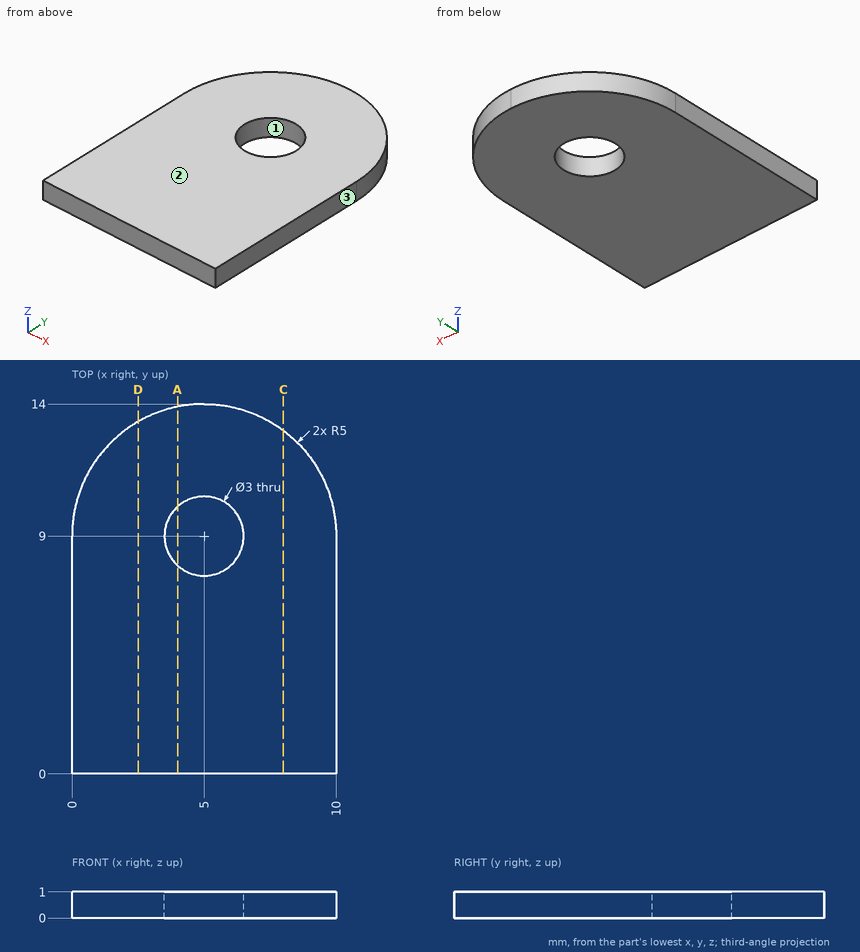
Study the drawing (mm; zero at the part's minimum x, y, z) and answer. Coordinates: 2 decimals unless noted, no trailing zeros. Loops run counter-clockwise (first coordinate to the right, second up) from the corner with the lowest first, then second, coordinate; pieces in that order, holes last. Notation, with made-up numbers: (20.25, 19) -> (63.25, 19) arc R12 cw to (63.25, 40) -> close; hole circle Ø3 at (42, 11). An arc over 180 degrees is marked (long way). Answer in a Markdown table with one row per item. Add a question column.
1. The part is cut by section A-A, the plane x = 4. Write down the section's boundary in (y, z).
2. The part is cut by section D-D, the plane x = 2.5. Write down the section's boundary in (y, z).
3. A flat-ended cylindrical pin translates along its axis: P1, Ø1.8, axis at x = 5, y = 9, coming from the -Z side. Find the tip coordinate at first contact, or state that the pin passes through.
4. Determine the mould class of the marked faces 1, 2 and 3 for opening direction X: +X half, -X half, draft (parallel to the pull), parting line (faces both ways), or undercut.
5. The part is cut by section C-C, the plane x = 8. Write down the section's boundary in (y, z), then the cut area to 3 significant figures.
6. Consider line 1 (Y direction, x = 5, z = 0.4); line 2 (X direction, y = 9, z = 0.3); line 3 (Y direction, x = 3.75, z = 0.7) (1 decimal). Determine where each line is inside the solid, lowest interval first. Write a range as [from, to].
Answer below:
| question | item | result |
|---|---|---|
| 1 | outline | (0, 0) -> (7.88, 0) -> (7.88, 1) -> (0, 1) -> close; (10.12, 0) -> (13.9, 0) -> (13.9, 1) -> (10.12, 1) -> close |
| 2 | outline | (0, 0) -> (13.33, 0) -> (13.33, 1) -> (0, 1) -> close |
| 3 | P1 | through |
| 4 | face 1 | undercut |
| 4 | face 2 | draft |
| 4 | face 3 | +X half |
| 5 | outline | (0, 0) -> (13, 0) -> (13, 1) -> (0, 1) -> close |
| 5 | area | 13.0 mm2 |
| 6 | line 1 | [0, 7.5], [10.5, 14] |
| 6 | line 2 | [0, 3.5], [6.5, 10] |
| 6 | line 3 | [0, 8.2], [9.8, 13.8] |
